Autodesk Inventor part; units mm, degrees
ref_plane "YZ Plane" through (0, 0, 0) normal (1, 0, 0) x (0, 1, 0)
ref_plane "XZ Plane" through (0, 0, 0) normal (0, 1, 0) x (-1, 0, 0)
ref_plane "XY Plane" through (0, 0, 0) normal (0, 0, 1) x (1, 0, 0)
ref_plane "Work Plane2" through (153.4386, -53.4776, -92.0146) normal (0, 0, -1) x (0, -1, 0)
sketch "Sketch2" plane through (153.4386, -53.4776, -92.0146) normal (0, 0, -1) x (0, -1, 0)
  line L0 (93.2, 97.5) -> (213.5, 97.5) construction
  line L1 (40, 105.5) -> (170, 105.5) construction
  line L2 (-3.5, 97.5) -> (93.2, 97.5) construction
  line L3 (40, 105.5) -> (170, 105.5) construction
  line L4 (0.0695, 95.5) -> (93.2, 95.5) construction
  line L5 (93.2, 95.5) -> (209.9305, 95.5) construction
  arc A0 (93.2, 56.229) -> (86.5748, 48.5) centre (107.9, 36.9243) ccw construction
  line L6 (93.2, 95.5) -> (93.2, 56.229) construction
  arc A1 (120.0681, 57.9171) -> (93.2, 56.229) centre (107.9, 36.9243) ccw construction
  arc A2 (128.5511, 49.6637) -> (120.0681, 57.9171) centre (125, 54.5) ccw construction
  arc A3 (129.2252, 48.5) -> (128.5511, 49.6637) centre (107.9, 36.9243) ccw construction
  line L7 (134.8038, 48.5) -> (129.2252, 48.5) construction
  arc A4 (145.1962, 48.5) -> (134.8038, 48.5) centre (140, 51.5) ccw construction
  line L8 (159.8038, 48.5) -> (145.1962, 48.5) construction
  arc A5 (170.1962, 48.5) -> (159.8038, 48.5) centre (165, 51.5) ccw construction
  line L9 (184.8038, 48.5) -> (170.1962, 48.5) construction
  arc A6 (195.1962, 48.5) -> (184.8038, 48.5) centre (190, 51.5) ccw construction
  line L10 (198.5, 48.5) -> (195.1962, 48.5) construction
  arc A7 (204.5, 42.5) -> (198.5, 48.5) centre (198.5, 42.5) ccw construction
  line L11 (204.5, -42.5) -> (204.5, 42.5)
  arc A8 (204.5, -42.5) -> (206.5, -44.5) centre (206.5, -42.5) ccw
  line L12 (207.3038, -44.5) -> (206.5, -44.5)
  arc A9 (215.5, -36.3038) -> (207.3038, -44.5) centre (212.5, -41.5) ccw
  line L13 (215.5, 87.3038) -> (215.5, -36.3038) construction
  arc A10 (207.3038, 95.5) -> (215.5, 87.3038) centre (212.5, 92.5) ccw construction
  line L14 (125, 95.5) -> (207.3038, 95.5) construction
  circle A11 centre (125, 89.5) radius 6 construction
  line L15 (93.2, 95.5) -> (125, 95.5) construction
  circle A12 centre (125, 72) radius 6 construction
  circle A13 centre (190, 76.5) radius 6 construction
  circle A14 centre (140, 76.5) radius 6 construction
  arc A15 (93.2, 53.646) -> (87.8, 46.5) centre (107.9, 36.9243) ccw construction
  arc A16 (128, 46.5) -> (93.2, 53.646) centre (107.9, 36.9243) ccw construction
  circle A17 centre (85, 89.5) radius 6 construction
  circle A18 centre (125, 89.5) radius 6 construction
  line L16 (79, 97.5) -> (79, 46.5)
  line L17 (79, 46.5) -> (87.8, 46.5)
  line L18 (79, 97.5) -> (131, 97.5)
  line L19 (131, 97.5) -> (131, 48.5)
  line L20 (131, 48.5) -> (131, 46.5)
  line L21 (131, 46.5) -> (128, 46.5)
  arc A19 (128, 46.5) -> (87.8, 46.5) centre (107.9, 36.9243) ccw
  circle A20 centre (85, 54.5) radius 1.95
  circle A21 centre (85, 72) radius 1.95
  circle A22 centre (85, 89.5) radius 1.95
  circle A23 centre (125, 89.5) radius 1.95
  circle A24 centre (125, 72) radius 1.95
  circle A25 centre (125, 54.5) radius 1.95
  point P0 (-53.4776, 153.4386)
extrude "Extrusion2" add sketch "Sketch2" along normal blind 5
shell "Shell2" thickness 2 removed faces 1 at (70.074, -152.3865, -97.0146)
properties part number "02_Zeiss_Axiotech_adapterplate_rightleft_connector"
Source: CAD feature listing. Evaluate the final solid. Frame: model axes, mm. A direction names the side the tool comes from. Give positions to 0.01 mm unless a question says otherwise; leave off trailing zeros. Loops run counter-clockwise (first coordinate to the right, second up) from the corner with the lowest first, then second, coordinate; pieces in that order, holes last. Notation, with made-up numbers: (75, 8) -> (81, 8) arc R12 ccw to (81, 27) -> close; hole circle Ø5 at (-2, 62). An arc over 180 degrees is marked (long way). Use a Markdown table: item, result. Add a question column.
(1) Access query for faces 1 (the face through (104.939, -137, -95)), 2 (the face through (66, -140, -97.015)). Directions: +Z, -Z, +X, -X, +Y, -Y. A direction counts if a zero-diameter tool reaches every point of the face in a straight line with its end or side. Return the directions, or none.
(2) Section query B-B (x = 80.5). Output: boundary loops of the cut face in (y, z), then the cut area to 3 significant figures.
(3) Section query C-C (x = 91). Output: boundary loops of the cut face in (y, z).
(4) First-contact query: pin 1 Ø2.5 at (x, y) = (63.94, -138.48) entering from -Z; pin 2 Ø1 at (y, z) = (-145, -96) entering from +X; pin 3 Ø5 at (x, y) = (81.44, -178.48) entering from +Z. Flat tips, straight axial feed; report the tip coordinate or a pass-through.
(5) Section query D-D (y = -166). Output: boundary loops of the cut face in (x, z), then the cut area to 3 significant figures.
(6) Section query A-A (z = -96.3). Count the separate pieces of the cut face and the enclosed holes in it, then the cut area to 3 significant figures.
(7) Ray query, line 1 (Y direction, x = 64, z = -93.6); line 2 (Y direction, x = 60.5, z = -95); line 3 (Y direction, x = 74, z = -95.8). Return the intervals inside material, ascending.
Checked values:
| question | item | result |
|---|---|---|
| 1 | face 1 | -Z |
| 1 | face 2 | -Z, +X, -X, +Y, -Y |
| 2 | outline | (-184.48, -97.01) -> (-182.48, -97.01) -> (-182.48, -94.01) -> (-182.31, -94.01) -> (-182.31, -97.01) -> (-180.19, -97.01) -> (-180.19, -92.01) -> (-184.48, -92.01) -> close; (-176.77, -97.01) -> (-174.64, -97.01) -> (-174.64, -94.01) -> (-142.31, -94.01) -> (-142.31, -97.01) -> (-140.19, -97.01) -> (-140.19, -92.01) -> (-176.77, -92.01) -> close; (-136.77, -97.01) -> (-134.64, -97.01) -> (-134.64, -94.01) -> (-134.48, -94.01) -> (-134.48, -97.01) -> (-132.48, -97.01) -> (-132.48, -92.01) -> (-136.77, -92.01) -> close |
| 2 | area | 128 mm^2 |
| 3 | outline | (-184.48, -97.01) -> (-182.48, -97.01) -> (-182.48, -94.01) -> (-134.48, -94.01) -> (-134.48, -97.01) -> (-132.48, -97.01) -> (-132.48, -92.01) -> (-184.48, -92.01) -> close |
| 4 | pin 1 | through |
| 4 | pin 2 | x = 101.99 |
| 4 | pin 3 | z = -92.01 |
| 5 | outline | (55.94, -97.01) -> (57.94, -97.01) -> (57.94, -94.01) -> (92.69, -94.01) -> (92.69, -97.01) -> (94.74, -97.01) -> (94.74, -92.01) -> (55.94, -92.01) -> close |
| 5 | area | 89.7 mm^2 |
| 6 | separate pieces | 6 |
| 6 | enclosed holes | 7 |
| 6 | area | 616 mm^2 |
| 7 | line 1 | -184.48 to -180.43, -176.53 to -140.43, -136.53 to -132.48 |
| 7 | line 2 | -184.48 to -182.48, -180.42 to -176.53, -140.42 to -136.53, -134.48 to -132.48 |
| 7 | line 3 | -184.48 to -182.48, -134.48 to -132.48 |
